Read the model definition and answer for the solid it produces. Units are mm, in the model's axes. A direction names the side the tool comes from. Give positions to 0.01 mm unless a question says otherwise; leave off trailing zeros. Return JSON: item names as keys, results as strings.
```python
from build123d import *

# Parameters (mm, degrees)
ENL_V_MAT_EXTRU_1_DEPTH  = 205
ESQUISSE4_W              = 219.421497641
ESQUISSE4_H              = 186.787380576
ENL_V_MAT_EXTRU_2_DEPTH  = 241.082722882
COQUE2_T                 = -10
ENL_V_MAT_EXTRU_4_DEPTH  = 5
ENL_V_MAT_EXTRU_5_DEPTH  = 25
ENL_V_MAT_EXTRU_6_DEPTH  = 2.5
ENL_V_MAT_EXTRU_10_DEPTH = 15
ECHELLE1_SCALE           = 1.15
TROU_TARAUD_M32_D        = 2.5
TROU_TARAUD_M32_DEPTH    = 12.5
TROU_TARAUD_M32_TIP      = 0.751075774
TROU_TARAUD_M33_D        = 2.5
TROU_TARAUD_M33_DEPTH    = 12.5
TROU_TARAUD_M33_TIP      = 0.751075774
TROU_TARAUD_M35_D        = 2.5
TROU_TARAUD_M35_DEPTH    = 12.5
TROU_TARAUD_M35_TIP      = 0.751075774
ESQUISSE23_R             = 1.5
ENL_V_MAT_EXTRU_11_DEPTH = 40


with BuildPart() as part:
    # Esquisse1 → Révolution2 (revolve)
    with BuildSketch(Plane.XY):
        with BuildLine():
            Line((0.334149559, -92.625367455), (0.334149559, 171))
            ThreePointArc((0.334149559, 171), (43.341663836, 173.345331392), (83, 190.148998741))
            ThreePointArc((83, 190.148998741), (97.133928161, 161.990328143), (102, 130.86156331))
            add(Edge.make_bspline(
                [(102, 130.86156331), (103.479009077, 113.684745488), (71.205293421, 65.560678141), (110.707376512, 34.252457406), (109.358599643, 11.86156331)],
                knots=[0, 0, 0, 0, 0.406612523, 1, 1, 1, 1], degree=3))
            ThreePointArc((109.358599643, 11.86156331), (99.215374733, -47.500625433), (59.334149559, -92.625367455))
            Line((59.334149559, -92.625367455), (0.334149559, -92.625367455))
        make_face()
    revolve(axis=Axis((0.334149559, -92.625367455, 0), (0, 1, 0)))

    # Esquisse3 → Enlèv. mat.-Extru.1 (cut, symmetric)
    with BuildSketch(Plane(origin=(0, 0, 0), x_dir=(1, 0, 0), z_dir=(0, 1, 0))):
        with BuildLine():
            Line((-97.244399695, 50.050229554), (0.334149559, 0))
            Line((0.334149559, 0), (92.468194445, 59.480387742))
            ThreePointArc((92.468194445, 59.480387742), (5.778653928, -109.530617295), (-97.244399695, 50.050229554))
        make_face()
    extrude(amount=ENL_V_MAT_EXTRU_1_DEPTH, both=True, mode=Mode.SUBTRACT)

    # Esquisse4 → Enlèv. mat.-Extru.2 (cut, through all)
    with BuildSketch(Plane.XY):
        with Locations((-2.038050308, 104.768322833)):
            Rectangle(ESQUISSE4_W, ESQUISSE4_H)
    extrude(amount=-ENL_V_MAT_EXTRU_2_DEPTH, mode=Mode.SUBTRACT)

    # Coque2
    coque2_openings = [part.faces().sort_by_distance(p)[0] for p in [
        (41.688799169, -36.484898267, -26.697955102),
        (-43.464282683, -36.484897866, -22.465199622),
    ]]
    offset(amount=COQUE2_T, openings=coque2_openings, kind=Kind.INTERSECTION)

    # Esquisse6 → Enlèv. mat.-Extru.4 (cut)
    with BuildSketch(Plane(origin=(0, 11.5, 0), x_dir=(1, 0, 0), z_dir=(0, 1, 0))):
        with BuildLine():
            Line((-64.751451353, 33.383866548), (0.334149559, 0))
            Line((0.334149559, 0), (61.788226523, 39.673850536))
            ThreePointArc((61.788226523, 39.673850536), (-3.29737439, 73.057717085), (-64.751451353, 33.383866548))
        make_face()
    extrude(amount=-ENL_V_MAT_EXTRU_4_DEPTH, mode=Mode.SUBTRACT)

    # Esquisse7 → Enlèv. mat.-Extru.5 (cut)
    with BuildSketch(Plane(origin=(0, 11.5, 0), x_dir=(1, 0, 0), z_dir=(0, 1, 0))):
        with BuildLine():
            Line((-40.77485255, 21.085730501), (0.334149559, 0))
            Line((0.334149559, 0), (39.149428885, 25.0585749))
            ThreePointArc((39.149428885, 25.0585749), (-1.959573224, 46.144305401), (-40.77485255, 21.085730501))
        make_face()
    extrude(amount=-ENL_V_MAT_EXTRU_5_DEPTH, mode=Mode.SUBTRACT)

    # Esquisse8 → Enlèv. mat.-Extru.6 (cut, symmetric)
    with BuildSketch(Plane(origin=(0, -92.5, 0), x_dir=(1, 0, 0), z_dir=(0, 1, 0))):
        with BuildLine():
            Line((36.828161908, 23.559998993), (0.334149559, 0))
            Line((0.334149559, 0), (-38.316414256, 19.824742283))
            ThreePointArc((-38.316414256, 19.824742283), (-1.822401908, 43.384741276), (36.828161908, 23.559998993))
        make_face()
    extrude(amount=ENL_V_MAT_EXTRU_6_DEPTH, both=True, mode=Mode.SUBTRACT)

    # Esquisse10 → Enlèv. mat.-Extru.10 (cut)
    with BuildSketch(Plane(origin=(0, -92.5, 0), x_dir=(1, 0, 0), z_dir=(0, 1, 0))):
        with BuildLine():
            Line((-24.838107184, 12.911415859), (0.334149559, 0))
            Line((0.334149559, 0), (24.101892064, 15.344105881))
            ThreePointArc((24.101892064, 15.344105881), (-1.070364679, 28.25552174), (-24.838107184, 12.911415859))
        make_face()
    extrude(amount=ENL_V_MAT_EXTRU_10_DEPTH, mode=Mode.SUBTRACT)


with BuildPart() as part_1:
    # Echelle1: scaled about (-3.205196898, -32.62107135, -71.203315854)
    add(part.part.scale(ECHELLE1_SCALE).moved(Location((0.480779535, 4.893160702, 10.680497378))))

    # Trou taraudé M32
    with Locations(Plane(origin=(-21.564432755, -98.60683867, -24.05170562), x_dir=(0, 0, -1), z_dir=(0, -1, 0))):
        with Locations((0, 0), (2.053122984, 41.304003571)):
            Hole(TROU_TARAUD_M32_D / 2, depth=TROU_TARAUD_M32_DEPTH)
            with Locations((0, 0, -(TROU_TARAUD_M32_DEPTH + TROU_TARAUD_M32_TIP / 2))):  # 118° drill point
                Cone(0, TROU_TARAUD_M32_D / 2, TROU_TARAUD_M32_TIP, mode=Mode.SUBTRACT)

    # Trou taraudé M33
    with Locations(Plane(origin=(-45.802285112, 12.36816133, -39.635090601), x_dir=(0, 0, 1), z_dir=(0, 1, 0))):
        with Locations((0, 0), (-4.379976461, 88.114820569)):
            Hole(TROU_TARAUD_M33_D / 2, depth=TROU_TARAUD_M33_DEPTH)
            with Locations((0, 0, -(TROU_TARAUD_M33_DEPTH + TROU_TARAUD_M33_TIP / 2))):  # 118° drill point
                Cone(0, TROU_TARAUD_M33_D / 2, TROU_TARAUD_M33_TIP, mode=Mode.SUBTRACT)

    # Trou taraudé M35
    with Locations(Plane(origin=(82.53934023, 17.973988757, -47.019680031), x_dir=(1, 0, 0), z_dir=(0, 1, 0))):
        with Locations((0, 0), (-66.69965831, 41.172267137), (-114.254701281, 36.84355094)):
            Hole(TROU_TARAUD_M35_D / 2, depth=TROU_TARAUD_M35_DEPTH)
            with Locations((0, 0, -(TROU_TARAUD_M35_DEPTH + TROU_TARAUD_M35_TIP / 2))):  # 118° drill point
                Cone(0, TROU_TARAUD_M35_D / 2, TROU_TARAUD_M35_TIP, mode=Mode.SUBTRACT)

    # Esquisse23 → Enlèv. mat.-Extru.11 (cut)
    with BuildSketch(Plane(origin=(-19.273619273, -89.804688212, -82.066838873), x_dir=(-0.9876815415012294, 0.1155106334721785, 0.10555788048559506), z_dir=(-0.15647738679360396, -0.7291003694870504, -0.6662788294971496))):
        with Locations(Location((-10.604108873, 5.618400934, 0), (0, 0, 3.1152173))):
            Circle(ESQUISSE23_R)
        with Locations(Location((15.022911638, 1.230255574, 0), (0, 0, 2.971685795))):
            Circle(ESQUISSE23_R)
    extrude(amount=-ENL_V_MAT_EXTRU_11_DEPTH, mode=Mode.SUBTRACT)


solid = part_1.part
```
Q1. For faces 1 (the flat face through (-4, 17.974, -80)), 2 (the flat face through (90.75, -41.55, -47.35)), 3 (the flat face through (-2, -90.126, -29)), 4 (the cylindrical face through (-2.35, -100.1, -39.17)), 5 (the cylindrical face through (-2.08, 15.21, -73.39)), determine the directions among +Z, -Z, +X, -X, +Y, -Y from which every point of the face is accessible in a straight line to the end or side of a thin tool.
Values:
{"face 1": "+Z, -Z, +X, -X, +Y", "face 2": "+Z, +X, +Y, -Y", "face 3": "+Z", "face 4": "+Z, -Y", "face 5": "+Z, +Y"}
Q2. Given pin 1 (3 mm diameter, centred on x = -45.8, z = -39.64, fed in from +Y); pin 2 (2 mm diameter, centred on x = -31.72, z = -83.86, fed in from +Y); pin 3 (5 mm diameter, centred on x = 18, y = -13.5, fed in from +Z); pin 4 (2 mm diameter, centred on x = -21.56, z = -24.05, fed in from -Y), each flat-ended and moving along its own axis, determine where each tip first touches the part or whether it passes through.
Values:
{"pin 1": "stops at y = 12.37", "pin 2": "stops at y = -49.39", "pin 3": "stops at z = -100.56", "pin 4": "passes through"}
Q3. Determine the mould class of faces 6 (the flat face through (0, -98.607, -22)), 7 (the flat face through (-94.726, -37.117, -38.35)), 8 (the cylindrical face through (-7.294, -77.493, -76.678)) for opening direction Z: released by +Z, released by -Z, zero draft, split by the parting line, or undercut.
Values:
{"face 6": "zero draft", "face 7": "released by +Z", "face 8": "undercut"}
Q4. Consider L1, parallel to Y at x = 43.5, z = -26; L2, parallel to Y at x = 27, z = -13; L3, parallel to Y at x = -21.5, z = -58. Determine where each line is inside the solid, lowest interval first.
Values:
{"L1": "y = -101.63 to -90.13, 6.47 to 12.37", "L2": "y = -98.61 to -90.13", "L3": "y = -98.69 to -84.28, 6.47 to 12.37"}
